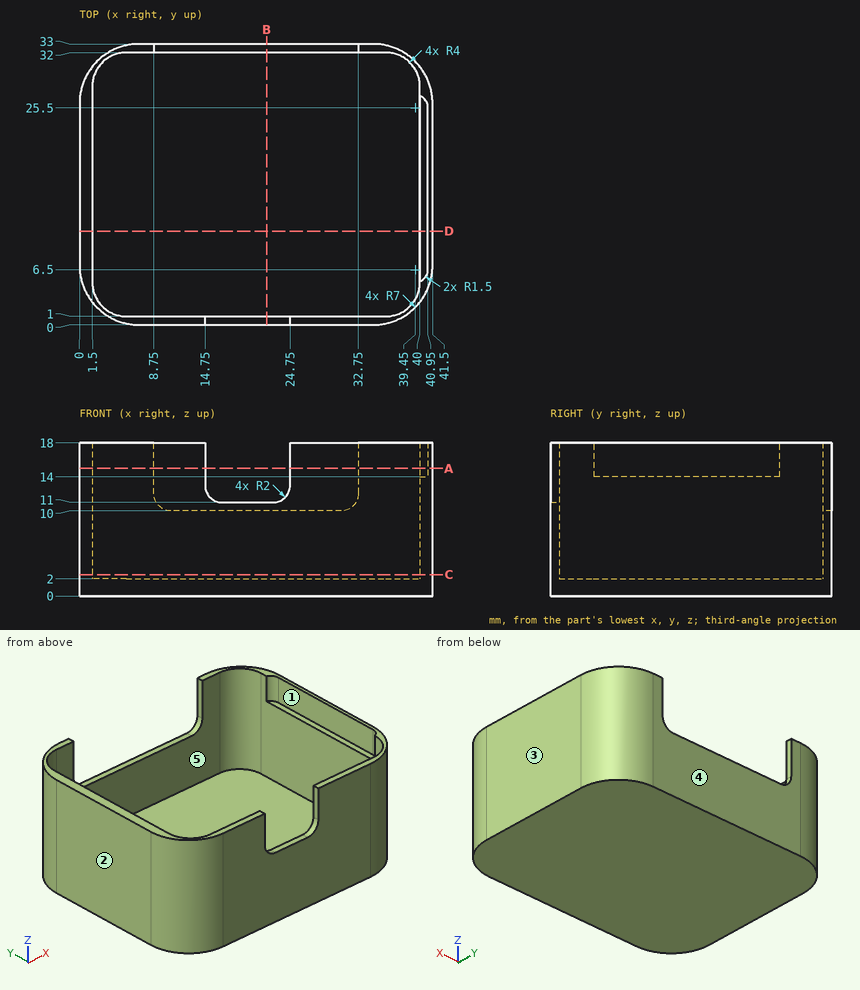
For this review, use the dimensioned drawing (mm, ordinates from the lowest corner) and the shaded views. A direction names the side the tool comes from. Give positions to 0.01 mm unless a question says otherwise; leave off trailing zeros. Write each loop counter-clockwise with the first axis right and the second up, starting at its lowest first coordinate (ties: lowest second). Pieces come first, ordered by that corner, then holes. Notation, with made-up numbers: M 18.5,21.25 L 55.5,21.25 A34 ccw 55.5,54.25 Z; hole C -7,10.25 d9. An arc over 180 degrees is marked long. Answer as a JSON object with one key per item and string values. Group by question number.
Item 1: Draft analysis for pull direction Y (two halves, no side actions). For the marked faces 3, 4 and 5, state which applies: +Y half, -Y half, draft (parallel to the pull), parting line (faces both ways), or undercut.
Item 2: Consider section A-A on z = 15. Write out the cut boundary in (x, y).
Item 3: Consider section C-C on z = 2.5. Write out the cut boundary in (x, y).
Item 4: Consider section D-D on y = 11. Write out the cut boundary in (x, z).
Item 5: For pin 1 Ø0.5 at (x, y) = (40.5, 15) entering from +Z; pin 2 Ø0.5 at (x, y) = (20.5, 32.5) entering from +Z; pin 3 Ø0.5 at (y, z) = (0.5, 15.5) entering from -X, all flat-tipped, find the tip position at first contact; note any pin that passes through.
Item 6: Consider section B-B on x = 22. Write out the cut boundary in (y, z), plus the area to 3 significant figures.
Item 7: For probe 1 along X at (y, z) = (16, 3.5); probe 2 along X at (y, z) = (10, 14.75); probe 3 along Y at (x, z) = (24, 3.5), list the stretches that pass through material, from the lowest coordinate up. Write a range as [from, to].
Item 8: Tool access review of the marked faces 1 and 2: name each direction out of +Z, -Z, +X, -X, +Y, -Y from which nothing blocks a thin tool from reaching the whole face with its end or side.
Check result:
{
 "1": {"face 3": "draft", "face 4": "+Y half", "face 5": "undercut"},
 "2": {"outline": "M 0,7 A7 ccw 7,0 L 14.75,0 L 14.75,1 L 5.5,1 A4 cw 1.5,5 L 1.5,28 A4 cw 5.5,32 L 8.75,32 L 8.75,33 L 7,33 A7 ccw 0,26 Z; M 24.75,0 L 34.5,0 A7 ccw 41.5,7 L 41.5,26 A7 ccw 34.5,33 L 32.75,33 L 32.75,32 L 36,32 A4 cw 40,28 L 40,26.9 A1.5 cw 40.95,25.5 L 40.95,6.5 A1.5 cw 40,5.1 L 40,5 A4 cw 36,1 L 24.75,1 Z"},
 "3": {"outline": "M 0,7 A7 ccw 7,0 L 34.5,0 A7 ccw 41.5,7 L 41.5,26 A7 ccw 34.5,33 L 7,33 A7 ccw 0,26 Z; hole M 1.5,5 A4 ccw 5.5,1 L 36,1 A4 ccw 40,5 L 40,28 A4 ccw 36,32 L 5.5,32 A4 ccw 1.5,28 Z"},
 "4": {"outline": "M 0,0 L 41.5,0 L 41.5,18 L 40.95,18 L 40.95,14 L 40,14 L 40,2 L 1.5,2 L 1.5,18 L 0,18 Z"},
 "5": {"pin 1": "stops at z = 14", "pin 2": "stops at z = 10", "pin 3": "stops at x = 3.85"},
 "6": {"outline": "M 0,0 L 33,0 L 33,10 L 32,10 L 32,2 L 1,2 L 1,11 L 0,11 Z", "area": "83.0 mm^2"},
 "7": {"probe 1": "x = [0, 1.5], [40, 41.5]", "probe 2": "x = [0, 1.5], [40.95, 41.5]", "probe 3": "y = [0, 1], [32, 33]"},
 "8": {"face 1": "+Z", "face 2": "+Z, -Z, -X, +Y, -Y"}
}
